```python
from build123d import *

# Parameters (mm, degrees)
F1_DEPTH = 3.81
F2_R     = 5.08
F3_R     = 865.118216
F4_R     = 162.209665


with BuildPart() as f1:
    # F0 (on Top) → F1 (new body)
    with BuildSketch(Plane.XY):
        with BuildLine():
            ThreePointArc((159.982175, -14.983156), (131.487989, -4.776084), (101.6, 0))
            ThreePointArc((101.6, 0), (50.8, 1.883753), (0, 0))
            ThreePointArc((0, 0), (0.527793, -5.453793), (0, -10.907586))
            ThreePointArc((0, -10.907586), (38.216498, -12.540312), (76.432995, -10.907586))
            ThreePointArc((76.432995, -10.907586), (97.285986, -8.193881), (117.188677, -14.983156))
            ThreePointArc((117.188677, -14.983156), (135.458144, -22.361969), (151.831031, -33.323213))
            ThreePointArc((151.831031, -33.323213), (157.950398, -25.061539), (159.982175, -14.983156))
        make_face()
    extrude(amount=F1_DEPTH)

    # F2
    f2_edges = [f1.edges().sort_by_distance(p)[0] for p in [
        (151.831031, -33.323213, 1.905),
        (159.982175, -14.983156, 1.905),
    ]]
    fillet(f2_edges, radius=F2_R)

    # F3
    f3_edges = [f1.edges().sort_by_distance(p)[0] for p in [
        (117.188677, -14.983156, 1.905),
    ]]
    fillet(f3_edges, radius=F3_R)

    # F4
    f4_edges = [f1.edges().sort_by_distance(p)[0] for p in [
        (76.432995, -10.907586, 1.905),
    ]]
    fillet(f4_edges, radius=F4_R)


solid = f1.part
```
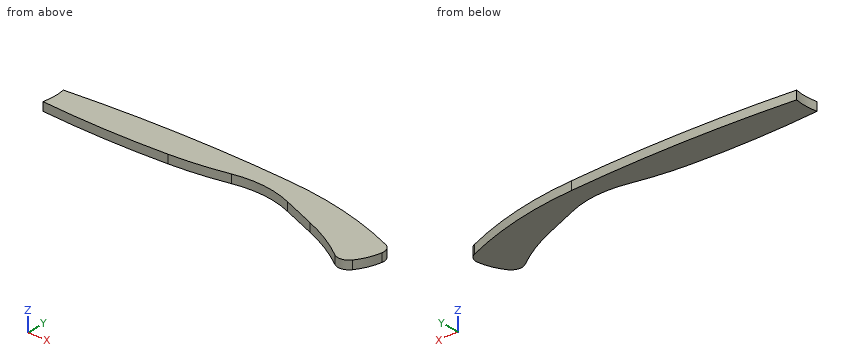
Geometry: final body of the model. Coordinates: model frame, mm. Round coordinates to 2 decimals unless told otherwise and drop trailing zeros. Order: outer loops, then holes, each group sorted by start corner. A loop starts at its lowest first (then second) coordinate and runs counter-clockwise, first axis right, second up. Notation, with made-up numbers: (16.25, 32) -> (34.25, 32) arc R15 cw to (34.25, 48) -> close; hole circle Ø2 at (54, 84.25). An arc over 180 degrees is marked (long way). Use CSV: the item, a comma, the result in double quotes. Start each with the question number.
1) Section A-A (x = 141). Return the cut outline in (y, z).
2) Section B-B (y = -3). Return the cut outline in (x, z), and give its area (3 significant figures).
3) First-contact query: pin 1 Ø8 at (x, y) = (53.5, -18.5) entering from +Z. Flat tip, straight axial feed; report the tip coordinate or a pass-through.
4) Material intervals for line 1 along Y through (x, z) = (122, 2.3); line 2 along X through (y, z) = (-14, 0.6); line 3 along Y through (x, z) = (93, 0.55), sorted ascending. Write a range as from..to.
Returned:
1,outline,"(-25.54, 0) -> (-7.53, 0) -> (-7.53, 3.81) -> (-25.54, 3.81) -> close"
2,outline,"(0.42, 0) -> (123.8, 0) -> (123.8, 3.81) -> (0.42, 3.81) -> close"
2,area,"470 mm²"
3,pin 1,"passes through"
4,line 1,"y = -16.36..-2.64"
4,line 2,"x = 116.33..157.61"
4,line 3,"y = -7.97..0.58"
